Here's how the part is built. I have some questions about the finished solid (model axes, mm). Coordinates: 2 decimals unless noted, no trailing zeros. Write each loop counter-clockwise with the first axis right and the second up, starting at its lowest first coordinate (ties: lowest second). Pieces come first, ordered by that corner, then holes. Notation, with made-up numbers: (82, 76) -> (138, 76) arc R18 cw to (138, 87) -> close; hole circle Ø6 at (49, 60.25). An arc over 180 degrees is marked (long way). Use a Markdown table: item, result. Add a question column.
Item 1: If we mould it in two halves opening along X, with no side actions, what happens to faces 1 (the cylindrical face through (-9.197, 17.93, -2.552)), 2 (the flat face through (-17, 23, 0)), 3 (the flat face through (-34.6, 6, 1))? For each: pulls with the +X half, pulls with the -X half, needs draft (parallel to the pull), parting line crosses it, or undercut.
Item 2: Imagine slicing it at D-D, the plane z = 1.5. Write out the boundary of the cut face in (x, y), and give its area (3 significant figures).
Item 3: Imagine slicing it at A-A, the plane x = -17.3. Write out the boundary of the cut face in (y, z) (3 decimals), and give its area (3 significant figures).
Item 4: Imagine slicing it at C-C, the plane z = -36.5. Write out the boundary of the cut face in (x, y).
Item 5: Will this pin go through, and if not, where does the flat tip stop? pin 1 Ø21 at (x, z) = (1, 31.5) entering from +Y.
Item 6: Imagine slicing it at B-B, the plane y = 16.5. Write out the boundary of the cut face in (x, z) (3 decimals).
Item 7: If I drill on line 1 along Y through (x, z) = (-10.5, 13.5); line 2 along X through (y, z) = (15, 1.5); line 3 along Z through (x, y) = (-17, 21), over which ranges is the centre line in solid material (lowest first)? Write a range as from..to.
```python
from build123d import *

# Parameters (mm, degrees)
SKETCH1_W           = 69.2
SKETCH1_H           = 150.88406761
BOSS_EXTRUDE1_DEPTH = 13
BOSS_EXTRUDE2_DEPTH = 10


with BuildPart() as part:
    # Sketch1 → Boss-Extrude1 (new body)
    with BuildSketch(Plane(origin=(0, 0, 0), x_dir=(1, 0, 0), z_dir=(0, 1, 0))):
        Rectangle(SKETCH1_W, SKETCH1_H)
    extrude(amount=BOSS_EXTRUDE1_DEPTH)

    # Sketch2 → Boss-Extrude2 (add)
    with BuildSketch(Plane(origin=(0, 13, 0), x_dir=(1, 0, 0), z_dir=(0, 1, 0))):
        with BuildLine():
            ThreePointArc((-25.795, 0), (-17.3, -8.495), (-8.805, 0))
            Line((-8.805, 0), (-25.795, 0))
        make_face()
        with BuildLine():
            Line((-25.795, 0), (-8.805, 0))
            ThreePointArc((-8.805, 0), (-17.3, 8.495), (-25.795, 0))
        make_face()
        with BuildLine():
            ThreePointArc((25.820118221, 0.00925204), (17.327393087, 8.504251736), (8.83011944, 0.013801772))
            Line((8.83011944, 0.013801772), (25.820117003, 0.004702309))
            ThreePointArc((25.820117003, 0.004702309), (25.820117917, 0.006977175), (25.820118221, 0.00925204))
        make_face()
        with BuildLine():
            Line((25.820117003, 0.004702309), (8.83011944, 0.013801772))
            ThreePointArc((8.83011944, 0.013801772), (17.32056849, -8.485746741), (25.820117003, 0.004702309))
        make_face()
    extrude(amount=BOSS_EXTRUDE2_DEPTH)


solid = part.part
```
Ans:
| question | item | result |
|---|---|---|
| 1 | face 1 | undercut |
| 1 | face 2 | needs draft |
| 1 | face 3 | pulls with the -X half |
| 2 | outline | (-34.6, 0) -> (34.6, 0) -> (34.6, 13) -> (25.68, 13) -> (25.68, 23) -> (8.97, 23) -> (8.97, 13) -> (-8.94, 13) -> (-8.94, 23) -> (-25.66, 23) -> (-25.66, 13) -> (-34.6, 13) -> close |
| 2 | area | 1,230 mm^2 |
| 3 | outline | (0, -75.442) -> (13, -75.442) -> (13, -8.495) -> (23, -8.495) -> (23, 8.495) -> (13, 8.495) -> (13, 75.442) -> (0, 75.442) -> close |
| 3 | area | 2,130 mm^2 |
| 4 | outline | (-34.6, 0) -> (34.6, 0) -> (34.6, 13) -> (-34.6, 13) -> close |
| 5 | pin 1 | stops at y = 13 |
| 6 | outline | circle Ø16.99 at (-17.3, 0); (25.82, -0.009) arc R8.484 ccw to (25.82, -0.005) arc R8.495 ccw (long way) to start |
| 7 | line 1 | y = 0..13 |
| 7 | line 2 | x = -25.66..-8.94, 8.97..25.68 |
| 7 | line 3 | z = -8.49..8.49 |
